Can you work these out from the model? Positions are in its coordinate system, mm. Give positions to 0.01 mm unless a question says otherwise; leave off trailing zeros. Order: outer loops, then holes, each group sorted by start corner. A loop starts at its lowest first (then second) coordinate and runs counter-clockwise, first axis right, second up. Notation, with made-up numbers: (65.5, -2) - (92.5, -2) arc R17 cw to (92.5, 29) - close; hole circle Ø8 at (86.25, 61). An arc over 180 degrees is marked (long way). Return JSON: item names as keys, results as strings.
```python
from build123d import *

# Parameters (mm, degrees)
F0_R     = 4
F1_DEPTH = 63.5
F3_ANGLE = 30
F4_W     = 20
F4_H     = 20
F5_DEPTH = 4.001


with BuildPart() as f1:
    # F0 (on Front) → F1 (new body)
    with BuildSketch(Plane.XZ):
        with Locations((0, 4)):
            Circle(F0_R)
    extrude(amount=-F1_DEPTH)


with BuildPart() as f1_1:
    # F3: moved
    add(f1.part.rotate(Axis((2.8749, 0, 0), (1, 0, 0)), F3_ANGLE))

    # F4 (on Front) → F5 (cut, through all)
    with BuildSketch(Plane.XZ):
        Rectangle(F4_W, F4_H)
    extrude(amount=F5_DEPTH, mode=Mode.SUBTRACT)


solid = f1_1.part
```
1. For pin 1 Ø1 at (y, z) = (18, 15.5) entering from -X; pin 2 Ø2 at (x, y) = (-1.5, 16.5) entering from -Z; pin 3 Ø1 at (x, y) = (0.5, 33.5) entering from +Z; pin 4 Ø1 at (y, z) = (36, 23.5) entering from -X, each with a flat end and sliding along its axis, tell me the tip position at first contact or that it passes through.
Checks:
{"pin 1": "x = -4", "pin 2": "z = 9.17", "pin 3": "z = 28.84", "pin 4": "x = -3.83"}
2. Thinking about a two-plate mould opening in Y: for faces 1 (the face through (-0.056, 52.965, 35.263)), 2 (the face through (0, 0, 5)), 3 (the face through (-0.867, 27.064, 15.735)), which applies, +Y half, -Y half, draft (parallel to the pull), parting line (faces both ways), or undercut?
Checks:
{"face 1": "+Y half", "face 2": "-Y half", "face 3": "parting line"}
3. Suppose I cut it at B-B (x = -2.25). List the corners of the cut face in (y, z) for me, plus the area to 3 significant figures.
Checks:
{"outline": "(0, 0.8) - (54.65, 32.35) - (51.34, 38.08) - (0, 8.44) - close", "area": "405 mm^2"}
4. If I drill on L1, parallel to Z at x = 2.5, y = 35.5; L2, parallel to Z at x = -1.25, y = 48; L3, parallel to Y at x = -0.5, z = 28, over which ranges is the centre line in solid material (lowest first)? Write a range as [from, to].
Checks:
{"L1": "[21.51, 28.72]", "L2": "[27.94, 36.72]", "L3": "[32.56, 48.43]"}
5. Suppose I cut it at A-A (x = 1.75). List the corners of the cut face in (y, z) for me.
Checks:
{"outline": "(0, 0.47) - (54.79, 32.1) - (51.19, 38.33) - (0, 8.77) - close"}
